The model under review builds one solid part; all positions refer to its coordinate system, in mm. Round coordinates to 2 decimals unless told otherwise and drop trailing zeros. Order: outer loops, then holes, each group sorted by start corner. A loop starts at its lowest first (then second) coordinate and runs counter-clockwise, first axis right, second up. Notation, with made-up numbers: M 70,-3.75 L 78,-3.75 A19 cw 78,20.25 Z; hole C 48,38 d8. An arc over 180 degrees is marked long. Answer as CSV lines item,"result". Start each with the question number.
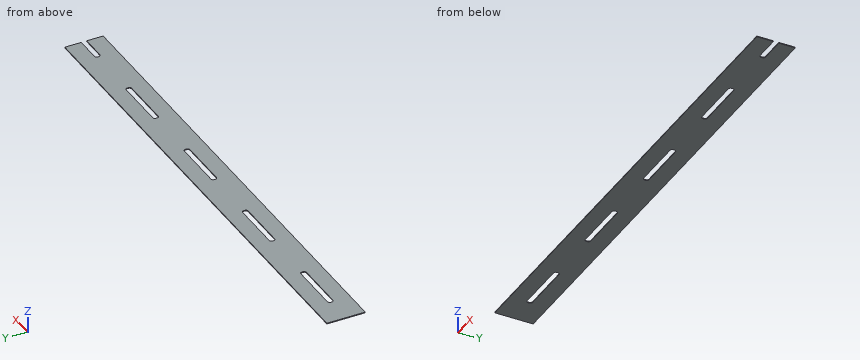
from build123d import *

# Parameters (mm, degrees)
F1_DEPTH = 0.15


with BuildPart() as f1:
    # F0 (on Top) → F1 (new body)
    with BuildSketch(Plane.XY):
        with BuildLine():
            Line((70.7, -0.5), (70.7, -3.5))
            Line((70.7, -3.5), (80.8, -3.5))
            Line((80.8, -3.5), (90.9, -3.5))
            Line((90.9, -3.5), (90.9, -0.5))
            Line((90.9, -0.5), (86.3, -0.5))
            ThreePointArc((86.3, -0.5), (86.017157, -0.382843), (85.9, -0.1))
            Line((85.9, -0.1), (85.9, 0.1))
            ThreePointArc((85.9, 0.1), (86.017157, 0.382843), (86.3, 0.5))
            Line((86.3, 0.5), (90.9, 0.5))
            Line((90.9, 0.5), (90.9, 3.5))
            Line((90.9, 3.5), (80.8, 3.5))
            Line((80.8, 3.5), (70.7, 3.5))
            Line((70.7, 3.5), (70.7, 0.5))
            Line((70.7, 0.5), (75.3, 0.5))
            ThreePointArc((75.3, 0.5), (75.582843, 0.382843), (75.7, 0.1))
            Line((75.7, 0.1), (75.7, -0.1))
            ThreePointArc((75.7, -0.1), (75.582843, -0.382843), (75.3, -0.5))
            Line((75.3, -0.5), (70.7, -0.5))
        make_face()
        with BuildLine():
            Line((10.1, -0.5), (10.1, -3.5))
            Line((10.1, -3.5), (20.2, -3.5))
            Line((20.2, -3.5), (30.3, -3.5))
            Line((30.3, -3.5), (30.3, -0.5))
            Line((30.3, -0.5), (25.7, -0.5))
            ThreePointArc((25.7, -0.5), (25.417157, -0.382843), (25.3, -0.1))
            Line((25.3, -0.1), (25.3, 0.1))
            ThreePointArc((25.3, 0.1), (25.417157, 0.382843), (25.7, 0.5))
            Line((25.7, 0.5), (30.3, 0.5))
            Line((30.3, 0.5), (30.3, 3.5))
            Line((30.3, 3.5), (20.2, 3.5))
            Line((20.2, 3.5), (10.1, 3.5))
            Line((10.1, 3.5), (10.1, 0.5))
            Line((10.1, 0.5), (14.7, 0.5))
            ThreePointArc((14.7, 0.5), (14.982843, 0.382843), (15.1, 0.1))
            Line((15.1, 0.1), (15.1, -0.1))
            ThreePointArc((15.1, -0.1), (14.982843, -0.382843), (14.7, -0.5))
            Line((14.7, -0.5), (10.1, -0.5))
        make_face()
        with BuildLine():
            Line((30.3, -0.5), (30.3, -3.5))
            Line((30.3, -3.5), (40.4, -3.5))
            Line((40.4, -3.5), (50.5, -3.5))
            Line((50.5, -3.5), (50.5, -0.5))
            Line((50.5, -0.5), (45.9, -0.5))
            ThreePointArc((45.9, -0.5), (45.617157, -0.382843), (45.5, -0.1))
            Line((45.5, -0.1), (45.5, 0.1))
            ThreePointArc((45.5, 0.1), (45.617157, 0.382843), (45.9, 0.5))
            Line((45.9, 0.5), (50.5, 0.5))
            Line((50.5, 0.5), (50.5, 3.5))
            Line((50.5, 3.5), (40.4, 3.5))
            Line((40.4, 3.5), (30.3, 3.5))
            Line((30.3, 3.5), (30.3, 0.5))
            Line((30.3, 0.5), (34.9, 0.5))
            ThreePointArc((34.9, 0.5), (35.182843, 0.382843), (35.3, 0.1))
            Line((35.3, 0.1), (35.3, -0.1))
            ThreePointArc((35.3, -0.1), (35.182843, -0.382843), (34.9, -0.5))
            Line((34.9, -0.5), (30.3, -0.5))
        make_face()
        with BuildLine():
            Line((50.5, -0.5), (50.5, -3.5))
            Line((50.5, -3.5), (60.6, -3.5))
            Line((60.6, -3.5), (70.7, -3.5))
            Line((70.7, -3.5), (70.7, -0.5))
            Line((70.7, -0.5), (66.1, -0.5))
            ThreePointArc((66.1, -0.5), (65.817157, -0.382843), (65.7, -0.1))
            Line((65.7, -0.1), (65.7, 0.1))
            ThreePointArc((65.7, 0.1), (65.817157, 0.382843), (66.1, 0.5))
            Line((66.1, 0.5), (70.7, 0.5))
            Line((70.7, 0.5), (70.7, 3.5))
            Line((70.7, 3.5), (60.6, 3.5))
            Line((60.6, 3.5), (50.5, 3.5))
            Line((50.5, 3.5), (50.5, 0.5))
            Line((50.5, 0.5), (55.1, 0.5))
            ThreePointArc((55.1, 0.5), (55.382843, 0.382843), (55.5, 0.1))
            Line((55.5, 0.1), (55.5, -0.1))
            ThreePointArc((55.5, -0.1), (55.382843, -0.382843), (55.1, -0.5))
            Line((55.1, -0.5), (50.5, -0.5))
        make_face()
        with BuildLine():
            Line((0, 3.5), (0, -3.5))
            Line((0, -3.5), (10.1, -3.5))
            Line((10.1, -3.5), (10.1, -0.5))
            Line((10.1, -0.5), (5.5, -0.5))
            ThreePointArc((5.5, -0.5), (5.217157, -0.382843), (5.1, -0.1))
            Line((5.1, -0.1), (5.1, 0.1))
            ThreePointArc((5.1, 0.1), (5.217157, 0.382843), (5.5, 0.5))
            Line((5.5, 0.5), (10.1, 0.5))
            Line((10.1, 0.5), (10.1, 3.5))
            Line((10.1, 3.5), (0, 3.5))
        make_face()
    extrude(amount=F1_DEPTH)


solid = f1.part
Item 1: Wall thickness on probe 1 along Y at (x, z) = (71, 0.1): over which ranges is the line inside the solid? List them lowest first. Write a range as [from, to].
Item 2: Consider section A-A (x = 8.5). State the section outline as (y, z) points, and give its area (3 significant figures).
Item 3: Consider section B-B (z = 0.1). State how many separate pieces and enclosed holes the cut face has, and give its area (3 significant figures).
Reported:
1,probe 1,"y = [-3.5, -0.5], [0.5, 3.5]"
2,outline,"M -3.5,0 L -0.5,0 L -0.5,0.15 L -3.5,0.15 Z; M 0.5,0 L 3.5,0 L 3.5,0.15 L 0.5,0.15 Z"
2,area,"0.900 mm²"
3,separate pieces,"1"
3,enclosed holes,"4"
3,area,"592 mm²"
